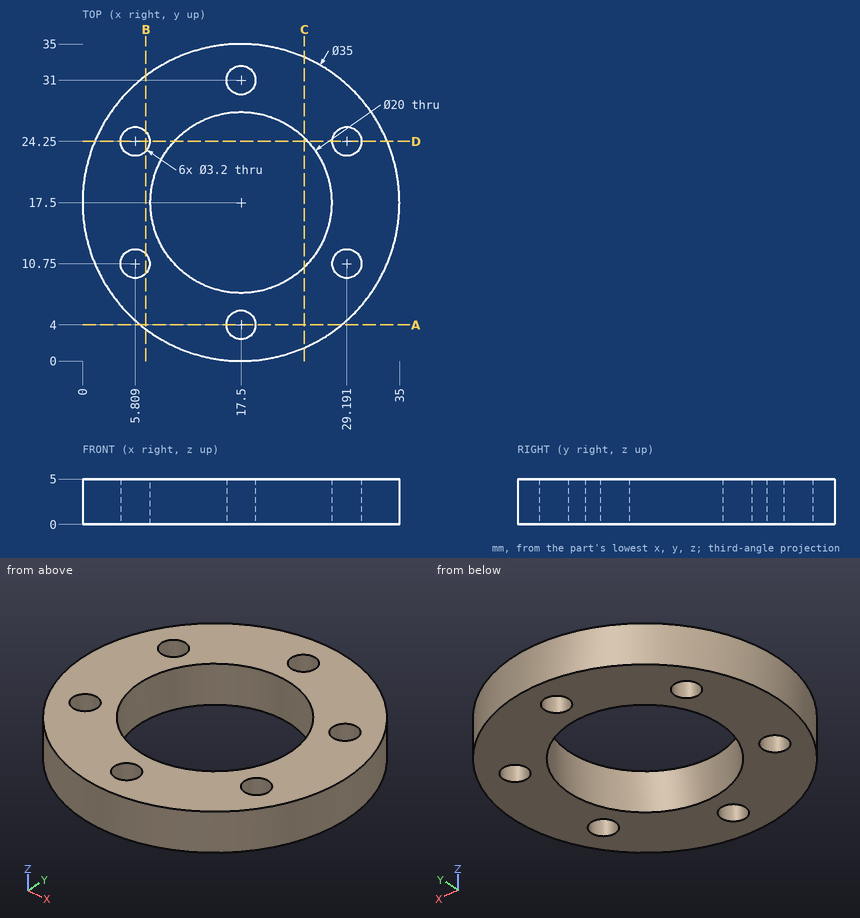
The figure shows three views and two pictorial views of one solid part (mm, origin at its lowest corner). Answer the questions. Give positions to 0.01 mm unless a question says otherwise; leave off trailing zeros. Order: outer loops, then holes, each group sorted by start corner. A loop starts at its lowest first (then second) coordinate and runs counter-clockwise, first axis right, second up. Notation, with made-up numbers: M -34,-10 L -6,-10 A26 ccw -6,25 Z; hole C -40,49.25 d6. An arc over 180 degrees is marked long. Return JSON: item names as keys, results as strings.
Q1. Find section C-C, the plane x = 24.5. Write down the section's boundary in (y, z).
Answer below:
{"outline": "M 1.46,0 L 10.36,0 L 10.36,5 L 1.46,5 Z; M 24.64,0 L 33.54,0 L 33.54,5 L 24.64,5 Z"}
Q2. Find section A-A, the plane y = 4. Write down the section's boundary in (x, z) (1 decimal).
Answer below:
{"outline": "M 6.4,0 L 15.9,0 L 15.9,5 L 6.4,5 Z; M 19.1,0 L 28.6,0 L 28.6,5 L 19.1,5 Z"}
Q3. Find section B-B, the plane x = 7. Write down the section's boundary in (y, z).
Answer below:
{"outline": "M 3.5,0 L 9.68,0 L 9.68,5 L 3.5,5 Z; M 11.82,0 L 23.18,0 L 23.18,5 L 11.82,5 Z; M 25.32,0 L 31.5,0 L 31.5,5 L 25.32,5 Z"}
Q4. Find the intervals of material crossed by line 1 along X through (y, z) = (24.5, 4.55); line 2 along Y through (x, z) = (30, 2.35); line 3 along Y through (x, z) = (17.5, 1.65), in increasing order. Write a range as [from, to].
Answer below:
{"line 1": "x = [1.46, 4.23], [7.39, 10.36], [24.64, 27.61], [30.77, 33.54]", "line 2": "y = [5.25, 9.37], [12.13, 22.87], [25.63, 29.75]", "line 3": "y = [0, 2.4], [5.6, 7.5], [27.5, 29.4], [32.6, 35]"}
Q5. Find section D-D, the plane y = 24.25. Write down the section's boundary in (x, z).
Answer below:
{"outline": "M 1.35,0 L 4.21,0 L 4.21,5 L 1.35,5 Z; M 7.41,0 L 10.12,0 L 10.12,5 L 7.41,5 Z; M 24.88,0 L 27.59,0 L 27.59,5 L 24.88,5 Z; M 30.79,0 L 33.65,0 L 33.65,5 L 30.79,5 Z"}
Q6. Each of these flat-tipped pins is pushed along its axis until it touches: pin 1 (1 mm diameter, centred on y = 14.5, z = 1, fed in from -X); pin 2 (2 mm diameter, centred on x = 22, z = 2, fed in from +Y); pin 3 (1.5 mm diameter, centred on y = 5.5, z = 1, fed in from -X) (1 decimal). Where does it stop, or does it pass through?
Answer below:
{"pin 1": "stops at x = 0.18", "pin 2": "stops at y = 34.65", "pin 3": "stops at x = 4.1"}
